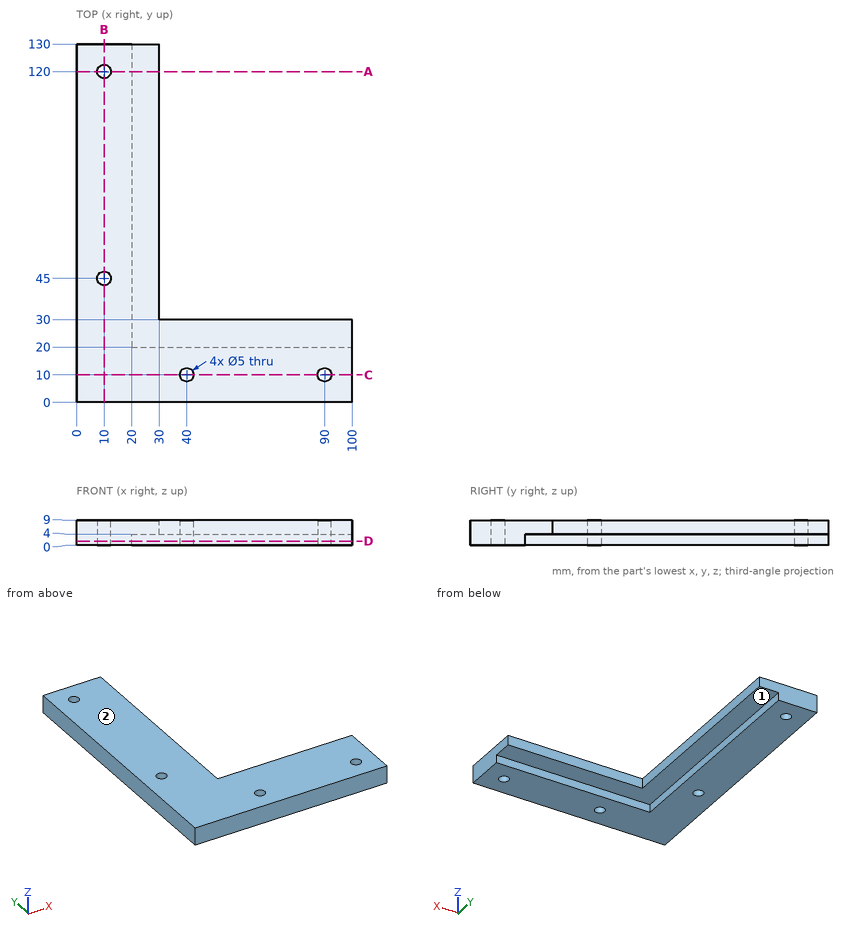
Check sheet for the drawn part. Datum: minimum x, y, z corner. Units: mm. A direction names the side the tool comes from. Coordinates: 2 decimals unless noted, no trailing zeros. Order: outer loops, then holes, each group sorted by start corner. A loop starts at its lowest first (then second) coordinate and runs counter-clockwise, first axis right, second up. Notation, with made-up numbers: M 49,70 L 68,70 A21 ccw 68,77 Z; hole C -27.75,54 d3. An arc over 180 degrees is marked long. One line per item, written item: value. Start each with the question number.
Item 1: Sectioned sample at C-C (y = 10). Enter the section's corners in (x, z), then the cut area to 3 significant figures.
Item 2: Sectioned sample at D-D (z = 1.5). Enter the section's corners in (x, y), then the cut area to 3 significant figures.
Item 3: Sectioned sample at B-B (x = 10). Enter the section's corners in (y, z).
Item 4: Access from +Z, -Z, +X, -X, +Y, -Y to the whole of each face (thin tool, end or side, straight path). Record for the marked faces 1 and 2.
Item 5: Sectioned sample at A-A (y = 120). Enter the section's corners in (x, z), then the cut area to 3 significant figures.
Item 6: Gauge pin test, flat ends, axial feed: pin 1 (5 mm diameter, centred on x = 41.5, z = 4, fed in from +Y); pin 2 (1.5 mm diameter, centred on y = 89, z = 7.5, fed in from +X); pin 3 (3 mm diameter, centred on y = 50.5, z = 1.5, fed in from +X). Record the tip position at first contact, or that the pin passes through.
Item 7: Scan lines: probe 1 along X at (y, z) = (10, 4.5); probe 2 along X at (y, z) = (45, 6); probe 3 along X at (y, z) = (120, 3.5). Record each from-to range of solid material in increasing order.
Conclusion:
1. outline: M 0,0 L 37.5,0 L 37.5,9 L 0,9 Z; M 42.5,0 L 87.5,0 L 87.5,9 L 42.5,9 Z; M 92.5,0 L 100,0 L 100,9 L 92.5,9 Z
1. area: 810 mm^2
2. outline: M 0,0 L 100,0 L 100,20 L 20,20 L 20,130 L 0,130 Z; hole C 10,45 d5; hole C 10,120 d5; hole C 40,10 d5; hole C 90,10 d5
2. area: 4,120 mm^2
3. outline: M 0,0 L 42.5,0 L 42.5,9 L 0,9 Z; M 47.5,0 L 117.5,0 L 117.5,9 L 47.5,9 Z; M 122.5,0 L 130,0 L 130,9 L 122.5,9 Z
4. face 1: -Z, +X, +Y
4. face 2: +Z, +X, -X, +Y, -Y
5. outline: M 0,0 L 7.5,0 L 7.5,9 L 0,9 Z; M 12.5,0 L 20,0 L 20,4 L 30,4 L 30,9 L 12.5,9 Z
5. area: 185 mm^2
6. pin 1: stops at y = 30
6. pin 2: stops at x = 30
6. pin 3: stops at x = 20
7. probe 1: x = 0 to 37.5, 42.5 to 87.5, 92.5 to 100
7. probe 2: x = 0 to 7.5, 12.5 to 30
7. probe 3: x = 0 to 7.5, 12.5 to 20
